Verification items for the finished model (mm, model axes). Coordinates: 2 decimals unless noted, no trailing zeros. Write each loop counter-clockwise with the first axis right and the second up, starting at its lowest first coordinate (ties: lowest second). Pieces come first, ordered by that corner, then holes. Notation, with made-up numbers: (-10, -19) -> (-6, -19) arc R24 ccw to (-6, 3) -> close; hole circle Ø1 at (19.5, 22). An arc over 180 degrees is marked (long way). Use a Markdown table: item, result. Add a question column.
from build123d import *

# Parameters (mm, degrees)
SKETCH1_W           = 210
SKETCH1_H           = 450
SKETCH1_W_2         = 150
SKETCH1_H_2         = 15
BOSS_EXTRUDE1_DEPTH = 6
SKETCH3_W           = 6
SKETCH3_H           = 24
BOSS_EXTRUDE3_DEPTH = 6
SKETCH2_W           = 24
SKETCH2_H           = 6
BOSS_EXTRUDE4_DEPTH = 6


with BuildPart() as part:
    # Sketch1 → Boss-Extrude1 (new body)
    with BuildSketch(Plane(origin=(0, 0, 0), x_dir=(1, 0, 0), z_dir=(0, 1, 0))):
        Rectangle(SKETCH1_W, SKETCH1_H)
        with Locations((0, -162.5)):
            Rectangle(SKETCH1_W_2, SKETCH1_H_2, mode=Mode.SUBTRACT)
        with Locations((0, -187.5)):
            Rectangle(SKETCH1_W_2, SKETCH1_H_2, mode=Mode.SUBTRACT)
        with Locations((0, -137.5)):
            Rectangle(SKETCH1_W_2, SKETCH1_H_2, mode=Mode.SUBTRACT)
        with Locations((0, -112.5)):
            Rectangle(SKETCH1_W_2, SKETCH1_H_2, mode=Mode.SUBTRACT)
        with Locations((0, -87.5)):
            Rectangle(SKETCH1_W_2, SKETCH1_H_2, mode=Mode.SUBTRACT)
        with Locations((0, -62.5)):
            Rectangle(SKETCH1_W_2, SKETCH1_H_2, mode=Mode.SUBTRACT)
        with Locations((0, -37.5)):
            Rectangle(SKETCH1_W_2, SKETCH1_H_2, mode=Mode.SUBTRACT)
        with Locations((0, -12.5)):
            Rectangle(SKETCH1_W_2, SKETCH1_H_2, mode=Mode.SUBTRACT)
        with Locations((0, 12.5)):
            Rectangle(SKETCH1_W_2, SKETCH1_H_2, mode=Mode.SUBTRACT)
        with Locations((0, 37.5)):
            Rectangle(SKETCH1_W_2, SKETCH1_H_2, mode=Mode.SUBTRACT)
        with Locations((0, 62.5)):
            Rectangle(SKETCH1_W_2, SKETCH1_H_2, mode=Mode.SUBTRACT)
        with Locations((0, 87.5)):
            Rectangle(SKETCH1_W_2, SKETCH1_H_2, mode=Mode.SUBTRACT)
        with Locations((0, 112.5)):
            Rectangle(SKETCH1_W_2, SKETCH1_H_2, mode=Mode.SUBTRACT)
        with Locations((0, 137.5)):
            Rectangle(SKETCH1_W_2, SKETCH1_H_2, mode=Mode.SUBTRACT)
        with Locations((0, 162.5)):
            Rectangle(SKETCH1_W_2, SKETCH1_H_2, mode=Mode.SUBTRACT)
        with Locations((0, 187.5)):
            Rectangle(SKETCH1_W_2, SKETCH1_H_2, mode=Mode.SUBTRACT)
    extrude(amount=BOSS_EXTRUDE1_DEPTH)

    # Sketch3 → Boss-Extrude3 (add)
    with BuildSketch(Plane(origin=(0, 6, 0), x_dir=(1, 0, 0), z_dir=(0, 1, 0))):
        with Locations((-108, 192)):
            Rectangle(SKETCH3_W, SKETCH3_H)
        with Locations((108, 192)):
            Rectangle(SKETCH3_W, SKETCH3_H)
        with Locations((108, 144)):
            Rectangle(SKETCH3_W, SKETCH3_H)
        with Locations((108, 96)):
            Rectangle(SKETCH3_W, SKETCH3_H)
        with Locations((108, 48)):
            Rectangle(SKETCH3_W, SKETCH3_H)
        with Locations((108, 0)):
            Rectangle(SKETCH3_W, SKETCH3_H)
        with Locations((108, -48)):
            Rectangle(SKETCH3_W, SKETCH3_H)
        with Locations((108, -96)):
            Rectangle(SKETCH3_W, SKETCH3_H)
        with Locations((108, -144)):
            Rectangle(SKETCH3_W, SKETCH3_H)
        with Locations((108, -192)):
            Rectangle(SKETCH3_W, SKETCH3_H)
        with Locations((-108, 144)):
            Rectangle(SKETCH3_W, SKETCH3_H)
        with Locations((-108, 96)):
            Rectangle(SKETCH3_W, SKETCH3_H)
        with Locations((-108, 48)):
            Rectangle(SKETCH3_W, SKETCH3_H)
        with Locations((-108, 0)):
            Rectangle(SKETCH3_W, SKETCH3_H)
        with Locations((-108, -48)):
            Rectangle(SKETCH3_W, SKETCH3_H)
        with Locations((-108, -96)):
            Rectangle(SKETCH3_W, SKETCH3_H)
        with Locations((-108, -144)):
            Rectangle(SKETCH3_W, SKETCH3_H)
        with Locations((-108, -192)):
            Rectangle(SKETCH3_W, SKETCH3_H)
    extrude(amount=-BOSS_EXTRUDE3_DEPTH)

    # Sketch2 → Boss-Extrude4 (add)
    with BuildSketch(Plane(origin=(0, 6, 0), x_dir=(1, 0, 0), z_dir=(0, 1, 0))):
        with Locations((-72, 228)):
            Rectangle(SKETCH2_W, SKETCH2_H)
        with Locations((-24, 228)):
            Rectangle(SKETCH2_W, SKETCH2_H)
        with Locations((24, 228)):
            Rectangle(SKETCH2_W, SKETCH2_H)
        with Locations((72, 228)):
            Rectangle(SKETCH2_W, SKETCH2_H)
        with Locations((-72, -228)):
            Rectangle(SKETCH2_W, SKETCH2_H)
        with Locations((-24, -228)):
            Rectangle(SKETCH2_W, SKETCH2_H)
        with Locations((24, -228)):
            Rectangle(SKETCH2_W, SKETCH2_H)
        with Locations((72, -228)):
            Rectangle(SKETCH2_W, SKETCH2_H)
    extrude(amount=-BOSS_EXTRUDE4_DEPTH)


solid = part.part
1) Cross-section at B-B on x = -19.5. Give the number of separate pieces and of enclosed holes in the cut face, then the cut area to 3 significant figures.
2) Thickness scan on L1, parallel to X at y = 0.4, z = 86.5; L2, parallel to X at y = 2.5, z = 16; L3, parallel to X at y = 4.2, z = -27.5. Record the ranges inside material, lowest first.
3) Cross-section at C-C on z = 162. Record the boundary of the cut face in (x, y), then the cut area to 3 significant figures.
4) Cross-section at A-A on z = -90. Record the boundary of the cut face in (x, y).
5) Gauge pin test, flat ends, axial feed: pin 1 (3 mm diameter, centred on y = 4.5, z = 114, fed in from +X); pin 2 (1.8 mm diameter, centred on x = 109.5, y = 3, fed in from -Z); pin 3 (1.8 mm diameter, centred on x = 91.5, y = 2.5, fed in from -Z); pin 4 (3 mm diameter, centred on x = 5.5, z = -127, fed in from -Y). Record the tip position at first contact, or that the pin passes through.
Returned:
| question | item | result |
|---|---|---|
| 1 | separate pieces | 17 |
| 1 | enclosed holes | 0 |
| 1 | area | 1,330 mm² |
| 2 | L1 | x = -111 to -75, 75 to 111 |
| 2 | L2 | x = -105 to -75, 75 to 105 |
| 2 | L3 | x = -105 to 105 |
| 3 | outline | (-105, 0) -> (-75, 0) -> (-75, 6) -> (-105, 6) -> close; (75, 0) -> (105, 0) -> (105, 6) -> (75, 6) -> close |
| 3 | area | 360 mm² |
| 4 | outline | (-111, 0) -> (-75, 0) -> (-75, 6) -> (-111, 6) -> close; (75, 0) -> (111, 0) -> (111, 6) -> (75, 6) -> close |
| 5 | pin 1 | stops at x = 105 |
| 5 | pin 2 | stops at z = -204 |
| 5 | pin 3 | stops at z = -225 |
| 5 | pin 4 | stops at y = 0 |
